Read the model definition and answer for the solid it produces. Units are mm, in the model's axes. Face numbers are marked on the shaded views. A direction names the side the tool comes from. Coordinates: 2 decimals unless noted, no trailing zeros. Write each loop counter-clockwise with the first axis right and the second up, starting at its lowest first coordinate (ties: lowest second). Pieces come first, ordered by that corner, then holes. Notation, with made-up numbers: M 0.25,75.5 L 41.25,75.5 A13 cw 41.25,98.5 Z; hole C 37.25,16.5 d1. An arc over 180 degrees is marked long. Use a Markdown table: item, result. Add a question column.
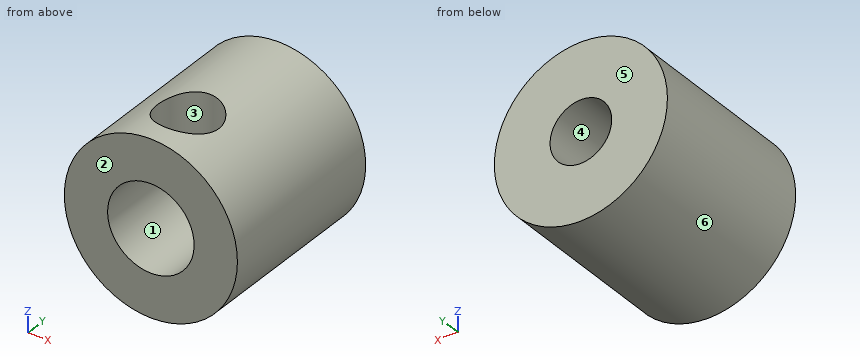
from build123d import *

# Parameters (mm, degrees)
SKETCH1_R                  = 3.175
BOSS_EXTRUDE1_DEPTH        = 6.5786
SKETCH2_R                  = 1.5875
CUT_EXTRUDE1_DEPTH         = 3.81
F_4_40_TAPPED_HOLE1_D      = 2.2606
F_4_40_TAPPED_HOLE1_DEPTH  = 12.7
F_4_40_TAPPED_HOLE1_TIP    = 0.679152758
F_4_40_TAPPED_HOLE2_REACH  = 11.679
F_4_40_TAPPED_HOLE2_BORE_R = 1.1303


with BuildPart() as part:
    # Sketch1 → Boss-Extrude1 (new body)
    with BuildSketch(Plane(origin=(0, 0, 0), x_dir=(1, 0, 0), z_dir=(0, 1, 0))):
        with Locations(Location((0, 0, 0), (0, 0, 270))):
            Circle(SKETCH1_R)
    extrude(amount=BOSS_EXTRUDE1_DEPTH)

    # Sketch2 → Cut-Extrude1 (cut)
    with BuildSketch(Plane.XZ):
        with Locations(Location((0, 0, 0), (0, 0, 270))):
            Circle(SKETCH2_R)
    extrude(amount=-CUT_EXTRUDE1_DEPTH, mode=Mode.SUBTRACT)

    # #4-40 Tapped Hole1
    with Locations(Plane(origin=(0, 6.5786, 0), x_dir=(1, 0, 0), z_dir=(0, 1, 0))):
        with Locations((0, 0)):
            Hole(F_4_40_TAPPED_HOLE1_D / 2, depth=F_4_40_TAPPED_HOLE1_DEPTH)
            with Locations((0, 0, -(F_4_40_TAPPED_HOLE1_DEPTH + F_4_40_TAPPED_HOLE1_TIP / 2))):  # 118° drill point
                Cone(0, F_4_40_TAPPED_HOLE1_D / 2, F_4_40_TAPPED_HOLE1_TIP, mode=Mode.SUBTRACT)

    # #4-40 Tapped Hole2 bore → #4-40 Tapped Hole2 (cut, up to next)
    with BuildSketch(Plane.XY.offset(3.175), mode=Mode.PRIVATE) as f_4_40_tapped_hole2_sk1:
        with Locations((0, 1.905)):
            Circle(F_4_40_TAPPED_HOLE2_BORE_R)
    f_4_40_tapped_hole2_tool1 = extrude(f_4_40_tapped_hole2_sk1.sketch, amount=-F_4_40_TAPPED_HOLE2_REACH, mode=Mode.PRIVATE) & part.part
    add(f_4_40_tapped_hole2_tool1.solids().sort_by_distance((0, 1.905, 3.175))[0], mode=Mode.SUBTRACT)


solid = part.part
Item 1: Consider probe 1 along Y at (x, z) = (0, 2); probe 2 along Z at (x, y) = (-2.75, 5.75); probe 3 along X at (y, z) = (2.25, 0) (1 decimal). Determine where each line is inside the solid, lowest interval first.
Item 2: Determine the mould class of the marked faces 4, 5 and 6 for opening direction Z: pulls with the +Z half, pulls with the -Z half, needs draft (parallel to the pull), parting line crosses it, or undercut.
Item 3: Find section A-A on x = 0. Give the vertices of the cut face in (y, z) (1 decimal).
Item 4: Find section D-D on z = -1. Give the vertices of the cut face in (x, y), then the cut area to 3 significant figures.
Item 5: For the marked faces 1, 2 and 3, determine the directions among +Z, -Z, +X, -X, +Y, -Y from which every point of the face is accessible in a straight line to the end or side of a thin tool.
Item 6: Find section B-B on z = 0. Give the vertices of the cut face in (x, y) (1 decimal).
Geometry says:
| question | item | result |
|---|---|---|
| 1 | probe 1 | y = 0 to 0.77, 3.04 to 6.58 |
| 1 | probe 2 | z = -1.59 to 1.59 |
| 1 | probe 3 | x = -3.2 to -1.6, 1.6 to 3.2 |
| 2 | face 4 | undercut |
| 2 | face 5 | needs draft |
| 2 | face 6 | parting line crosses it |
| 3 | outline | M 0,-3.2 L 6.6,-3.2 L 6.6,-1.1 L 3.8,-1.1 L 3.8,-1.6 L 0,-1.6 Z; M 0,1.6 L 0.8,1.6 L 0.8,3.2 L 0,3.2 Z; M 3,1.6 L 3.8,1.6 L 3.8,1.1 L 6.6,1.1 L 6.6,3.2 L 3,3.2 Z |
| 4 | outline | M -3.01,0 L -1.23,0 L -1.23,3.81 L -0.53,3.81 L -0.53,6.58 L -3.01,6.58 Z; M 0.53,3.81 L 1.23,3.81 L 1.23,0 L 3.01,0 L 3.01,6.58 L 0.53,6.58 Z |
| 4 | area | 27.3 mm2 |
| 5 | face 1 | -Y |
| 5 | face 2 | +Z, -Z, +X, -X, -Y |
| 5 | face 3 | +Z |
| 6 | outline | M -3.2,0 L -1.6,0 L -1.6,3.8 L -1.1,3.8 L -1.1,6.6 L -3.2,6.6 Z; M 1.1,3.8 L 1.6,3.8 L 1.6,0 L 3.2,0 L 3.2,6.6 L 1.1,6.6 Z |
